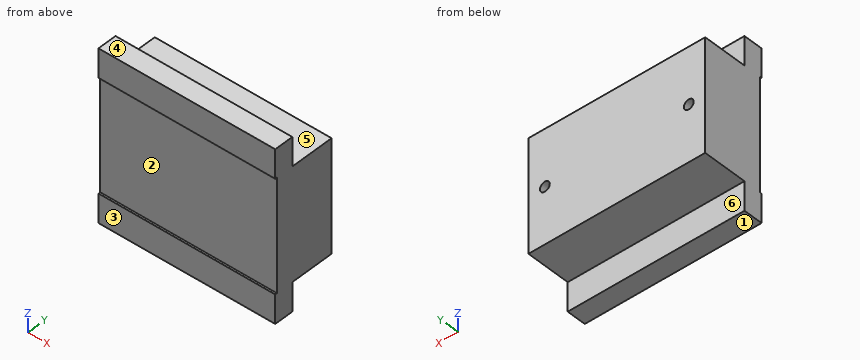
```python
from build123d import *

# Parameters (mm, degrees)
SKETCH1_W                   = 92.1
SKETCH1_H                   = 88.7
BOSS_EXTRUDE1_DEPTH         = 10
SKETCH2_W                   = 92.1
SKETCH2_H                   = 58.7
BOSS_EXTRUDE2_DEPTH         = 22.986
SKETCH16_W                  = 92.1
SKETCH16_H                  = 58.7
CUT_EXTRUDE2_DEPTH          = 1
F_1_4_20_TAPPED_HOLE1_D     = 5.1054
F_1_4_20_TAPPED_HOLE1_DEPTH = 16.51
F_1_4_20_TAPPED_HOLE1_TIP   = 1.533816902


with BuildPart() as part:
    # Sketch1 → Boss-Extrude1 (new body)
    with BuildSketch(Plane(origin=(0, 0, 0), x_dir=(1, 0, 0), z_dir=(0, 1, 0))):
        Rectangle(SKETCH1_W, SKETCH1_H)
    extrude(amount=BOSS_EXTRUDE1_DEPTH)

    # Sketch2 → Boss-Extrude2 (add)
    with BuildSketch(Plane(origin=(0, 10, 0), x_dir=(1, 0, 0), z_dir=(0, 1, 0))):
        Rectangle(SKETCH2_W, SKETCH2_H)
    extrude(amount=BOSS_EXTRUDE2_DEPTH)

    # Sketch16 → Cut-Extrude2 (cut)
    with BuildSketch(Plane.XZ):
        Rectangle(SKETCH16_W, SKETCH16_H)
    extrude(amount=-CUT_EXTRUDE2_DEPTH, mode=Mode.SUBTRACT)

    # 1/4-20 Tapped Hole1
    with Locations(Plane(origin=(0, 32.986, 0), x_dir=(-1, 0, 0), z_dir=(0, 1, 0))):
        with Locations((37.5, 0), (-37.5, 0)):
            Hole(F_1_4_20_TAPPED_HOLE1_D / 2, depth=F_1_4_20_TAPPED_HOLE1_DEPTH)
            with Locations((0, 0, -(F_1_4_20_TAPPED_HOLE1_DEPTH + F_1_4_20_TAPPED_HOLE1_TIP / 2))):  # 118° drill point
                Cone(0, F_1_4_20_TAPPED_HOLE1_D / 2, F_1_4_20_TAPPED_HOLE1_TIP, mode=Mode.SUBTRACT)


solid = part.part
```
Input: part model. Units: mm. Frame: model coordinates. Face numbers are marked on the shaded views. A direction names the side the tool comes from. Give positions to 0.01 mm unless a question says otherwise; leave off trailing zeros. Loops run counter-clockwise (first coordinate to the right, second up) from the corner with the lowest first, then second, coordinate; pieces in that order, holes last. Notation, with made-up numbers: M 6.5,68.5 L 45.5,68.5 A19 ccw 45.5,88.5 Z; hole C 28,-27.75 d10. An arc over 180 degrees is marked long. Answer as CSV lines item,"result". Start each with the question number.
1. Pin query (flat end, axial travel): P1, Ø4, axis at x = 34, y = 18.5, coming from the -Z side; P2, Ø4.5, axis at x = -8.5, z = -35.5, coming from the +Y side; P3, Ø7, axis at x = 3.5, y = 27, coming from the +Z side. Return the tip coordinate at first contact, or that it passes through.
2. Section A-A on x = -29.5. Return loops of the section in (y, z), plus the area to 3 significant figures.
3. Section C-C on z = 18. Return loops of the section in (x, y), plus the area to 3 significant figures.
4. Section B-B on y = 26.5. Return loops of the section in (x, z).
5. Line query: L1, parallel to X at y = 21.25, z = 0; L2, parallel to Z at x = -37.5, y = 26.75; L3, parallel to Y at x = 26, z = -11.5. Output: solid intervals per line, ascending.
6. Pull-direction query (Z, two-part tool) for the marked faces 1, 2 and 3; classes: released by +Z, released by -Z, zero draft, split by the parting line, or undercut.
7. Reachability of the marked faces 4, 5 and 6 from +Z, -Z, +X, -X, +Y, -Y: full face, straight path, thin tool, end or side. Return the list, or none.
Computed values:
1,P1,"stops at z = -29.35"
1,P2,"stops at y = 10"
1,P3,"stops at z = 29.35"
2,outline,"M 0,-44.35 L 10,-44.35 L 10,-29.35 L 32.99,-29.35 L 32.99,29.35 L 10,29.35 L 10,44.35 L 0,44.35 L 0,29.35 L 1,29.35 L 1,-29.35 L 0,-29.35 Z"
2,area,"2,180 mm²"
3,outline,"M -46.05,1 L 46.05,1 L 46.05,32.99 L -46.05,32.99 Z"
3,area,"2,950 mm²"
4,outline,"M -46.05,-29.35 L 46.05,-29.35 L 46.05,29.35 L -46.05,29.35 Z; hole C -37.5,0 d5.11; hole C 37.5,0 d5.11"
5,L1,"x = -46.05 to -40.05, -34.95 to 34.95, 40.05 to 46.05"
5,L2,"z = -29.35 to -2.55, 2.55 to 29.35"
5,L3,"y = 1 to 32.99"
6,face 1,"released by -Z"
6,face 2,"undercut"
6,face 3,"zero draft"
7,face 4,"+Z, +X, -X, +Y, -Y"
7,face 5,"+Z, +X, -X, +Y"
7,face 6,"-Z, +X, -X, +Y"
